Autodesk Inventor part; units mm, degrees
ref_plane "YZ Plane" through (0, 0, 0) normal (1, 0, 0) x (0, 1, 0)
ref_plane "XZ Plane" through (0, 0, 0) normal (0, 1, 0) x (-1, 0, 0)
ref_plane "XY Plane" through (0, 0, 0) normal (0, 0, 1) x (1, 0, 0)
sketch "Sketch1" plane through (0, 0, 0) normal (0, 0, 1) x (1, 0, 0)
  line L0 (0, 12.35) -> (250, 12.35)
  line L1 (0, 12.35) -> (0, 7.2)
  line L2 (0, 7.2) -> (250, 7.2)
  line L3 (250, 12.35) -> (250, 7.2)
  line L4 (250, 13.6) -> (0, 13.6)
  line L5 (0, -6.4) -> (250, -6.4)
  line L6 (250, -5.15) -> (0, -5.15)
  line L7 (250, 0) -> (250, -5.15)
  line L8 (0, 0) -> (250, 0)
  line L9 (0, 0) -> (0, -5.15)
  line L10 (250, -6.4) -> (220, -6.4)
  line L11 (220, -6.4) -> (220, 13.6)
  line L12 (220, 13.6) -> (250, 13.6)
  line L13 (250, 13.6) -> (250, -6.4)
  dimension "d0" = 30
extrude "Extrusion1" add sketch "Sketch1" along normal blind 6.35 contours L11 L4 L13 L0 | L0 L3 L2 L11 | L2 L13 L8 L11 | L8 L7 L6 L11 | L6 L13 L5 L11
sketch "Sketch2" plane through (0, 0, 6.35) normal (0, 0, 1) x (1, 0, 0)
  line L0 (250, 13.6) -> (220, 13.6)
  line L1 (220, -6.4) -> (250, -6.4)
  line L2 (220, 13.6) -> (250, -6.4)
  line L3 (235, 3.6) -> (250, 3.6)
  line L4 (250, -6.4) -> (250, 13.6)
  line L5 (235, 3.6) -> (220, 3.6)
  circle A0 centre (227.5, 3.6) radius 2.75
  circle A1 centre (242.5, 3.6) radius 2.75
  point P0 (0, 0)
  dimension "d3" = 5.5
extrude "Extrusion2" cut sketch "Sketch2" against normal blind 6.35 contours A0 L5 | L5 A0 | A1 L3 | L3 A1
sketch "Sketch3" plane through (0, 0, 6.35) normal (0, 0, 1) x (1, 0, 0)
  line L0 (220, -6.4) -> (220, 13.6)
  line L1 (220, -6.4) -> (224.604, -6.4)
  line L2 (224.604, -6.4) -> (224.604, -36.4)
  line L3 (224.604, -36.4) -> (220, -36.4)
  line L4 (220, -36.4) -> (220, -6.4)
  line L5 (250, -6.4) -> (220, -6.4)
  line L6 (233.2079, -6.4) -> (228.604, -6.4)
  line L7 (228.604, -6.4) -> (228.604, -36.4)
  line L8 (228.604, -36.4) -> (233.2079, -36.4)
  line L9 (233.2079, -36.4) -> (233.2079, -6.4)
  point P0 (0, 0)
  dimension "d6" = 30
  dimension "d7" = 4
extrude "Extrusion3" add sketch "Sketch3" against normal blind 6.35
sketch "Sketch4" plane through (0, 0, 6.35) normal (0, 0, 1) x (1, 0, 0)
  line L0 (233.2079, -6.4) -> (233.2079, -36.4)
  line L1 (233.2079, -36.4) -> (220, -36.4)
  line L2 (220, -36.4) -> (220, -42.75)
  line L3 (220, -42.75) -> (233.2079, -42.75)
  line L4 (233.2079, -42.75) -> (233.2079, -36.4)
  point P0 (0, 0)
  dimension "d10" = 6.35
extrude "Extrusion4" add sketch "Sketch4" against normal blind 6.35
sketch "Sketch5" plane through (0, 0, 0) normal (0, 0, -1) x (-1, 0, 0)
  line L0 (-228.604, -36.4) -> (-228.604, -6.4)
  line L1 (-228.604, -6.4) -> (-224.604, -6.4)
  line L2 (-224.604, -6.4) -> (-224.604, -36.4)
  line L3 (-224.604, -36.4) -> (-228.604, -36.4)
  circle A0 centre (-242.5, 3.6) radius 2.75
  circle A1 centre (-227.5, 3.6) radius 2.75
  line L4 (-233.2079, -6.4) -> (-233.2079, -42.75)
  line L5 (-233.2079, -42.75) -> (-220, -42.75)
  line L6 (-220, -42.75) -> (-220, 13.6)
  line L7 (-220, 13.6) -> (-250, 13.6)
  line L8 (-250, 13.6) -> (-250, -6.4)
  line L9 (-250, -6.4) -> (-233.2079, -6.4)
  line L10 (-233.2079, -6.4) -> (-233.2079, -42.75)
  line L11 (-233.2079, -6.4) -> (-220, -6.4)
  point P0 (0, 0)
extrude "Extrusion5" add sketch "Sketch5" along normal blind 6.35 contours L11 L9 L8 L7 L6 L1
properties part number "limitHolder"
Geometry check sheet. Reference: the model listing, model coordinates, mm. A direction names the side the tool comes from. Give positions to 0.01 mm unless a question says otherwise; leave off trailing zeros. Order: outer loops, then holes, each group sorted by start corner. A loop starts at its lowest first (then second) coordinate and runs counter-clockwise, first axis right, second up. Notation, with made-up numbers: (13, -4) - (27, -4) arc R20 cw to (27, 25) - close; hole circle Ø8 at (37, 41.5). An arc over 180 degrees is marked (long way). Answer in a Markdown table with one row per item. Add a question column.
Q1. Tool access check on faces 5 (the flat face through (233.208, -25, 3)), 6 (the flat face through (224.604, -21, 3)), 7 (the flat face through (231, -8, 6.35)). Record the directions out of +Z, -Z, +X, -X, +Y, -Y that give a thin tool (end or side, any length) a straight path to the whole face; none if there is none.
Q2. Mould release check, pull along Y, two halves, no side actions. Record for faces 1 (the cylindrical face through (242.681, 6.344, 0.089)), 2 (the flat face through (235, 13.6, 0)), 3 (the flat face through (224, -24, 0)), 4 (the flat face through (227, -42.75, 3)): pulls with the +Y half, pulls with the -Y half, needs draft (parallel to the pull), parting line crosses it, or undercut.
Q3. Material ranges on probe 1 along X at (y, z) = (3.6, 5.25); probe 2 along X at (y, z) = (-25, 5.5); probe 3 along Y at (x, z) = (227.5, -1.5), recorded low to high. Write a range as from..to.
Q4. Cross-section at B-B, the plane z = 4.25. Enter the section's corners in (x, y), then the cut area to 3 significant figures.
Q5. Cross-section at D-D, the plane x = 227.5. Enter the section's corners in (y, z), then the cut area to 3 significant figures.
Q6. Cross-section at C-C, the plane y = -30. Enter the section's corners in (x, z), then the cut area to 3 significant figures.
Q7. Gauge pin test, flat ends, axial feed: pin 1 (6 mm diameter, centred on x = 229, y = -34.5, fed in from -Z); pin 2 (1.9 mm diameter, centred on y = -28.5, z = 4.5, fed in from +X); pin 3 (1.5 mm diameter, centred on x = 224, z = -4, fed in from -Y). Record the tip position at first contact, or that the pin passes through.
Q8. Cross-section at A-A, the plane x = 242.5. Enter the section's corners in (y, z).
Check values:
| question | item | result |
|---|---|---|
| 1 | face 5 | +Z, -Z, +X, -Y |
| 1 | face 6 | +Z, -Z |
| 1 | face 7 | +Z, +X, -X, +Y, -Y |
| 2 | face 1 | undercut |
| 2 | face 2 | pulls with the +Y half |
| 2 | face 3 | needs draft |
| 2 | face 4 | pulls with the -Y half |
| 3 | probe 1 | x = 220..224.75, 230.25..239.75, 245.25..250 |
| 3 | probe 2 | x = 220..224.6, 228.6..233.21 |
| 3 | probe 3 | y = -6.4..0.85, 6.35..13.6 |
| 4 | outline | (220, -42.75) - (233.21, -42.75) - (233.21, -6.4) - (250, -6.4) - (250, 13.6) - (220, 13.6) - close; hole (224.6, -36.4) - (228.6, -36.4) - (228.6, -6.4) - (224.6, -6.4) - close; hole circle Ø5.5 at (227.5, 3.6); hole circle Ø5.5 at (242.5, 3.6) |
| 4 | area | 913 mm^2 |
| 5 | outline | (-42.75, 0) - (-36.4, 0) - (-36.4, 6.35) - (-42.75, 6.35) - close; (-6.4, -6.35) - (0.85, -6.35) - (0.85, 6.35) - (-6.4, 6.35) - close; (6.35, -6.35) - (13.6, -6.35) - (13.6, 6.35) - (6.35, 6.35) - close |
| 5 | area | 224 mm^2 |
| 6 | outline | (220, 0) - (224.6, 0) - (224.6, 6.35) - (220, 6.35) - close; (228.6, 0) - (233.21, 0) - (233.21, 6.35) - (228.6, 6.35) - close |
| 6 | area | 58.5 mm^2 |
| 7 | pin 1 | stops at z = 0 |
| 7 | pin 2 | stops at x = 233.21 |
| 7 | pin 3 | stops at y = -6.4 |
| 8 | outline | (-6.4, -6.35) - (0.85, -6.35) - (0.85, 6.35) - (-6.4, 6.35) - close; (6.35, -6.35) - (13.6, -6.35) - (13.6, 6.35) - (6.35, 6.35) - close |
